Geometry check sheet. Reference: the model listing, model coordinates, mm. A direction names the side the tool comes from. Round coordinates to 2 decimals unless told otherwise and drop trailing zeros. Loops run counter-clockwise (first coordinate to the right, second up) from the corner with the lowest first, then second, coordinate; pieces in that order, holes last.
```python
from build123d import *

# Parameters (mm, degrees)
BOSS_EXTRUDE1_DEPTH = 190
SHELL1_T            = -2
SKETCH3_R           = 17.5
CUT_EXTRUDE2_DEPTH  = 61


with BuildPart() as part:
    # Sketch1 → Boss-Extrude1 (new body, symmetric)
    with BuildSketch(Plane(origin=(0, 0, 0), x_dir=(1, 0, 0), z_dir=(0, 1, 0))):
        with BuildLine():
            Line((-24, -30), (24, -30))
            ThreePointArc((24, -30), (28.242640687, -28.242640687), (30, -24))
            Line((30, -24), (30, 24))
            ThreePointArc((30, 24), (28.242640687, 28.242640687), (24, 30))
            Line((24, 30), (-24, 30))
            ThreePointArc((-24, 30), (-28.242640687, 28.242640687), (-30, 24))
            Line((-30, 24), (-30, -24))
            ThreePointArc((-30, -24), (-28.242640687, -28.242640687), (-24, -30))
        make_face()
    extrude(amount=BOSS_EXTRUDE1_DEPTH, both=True)

    # Shell1
    shell1_openings = [part.faces().sort_by_distance(p)[0] for p in [
        (0, 190, 0),
        (0, -190, 0),
    ]]
    offset(amount=SHELL1_T, openings=shell1_openings, kind=Kind.INTERSECTION)

    # Sketch3 → Cut-Extrude2 (cut, through all)
    with BuildSketch(Plane(origin=(0, 0, -30), x_dir=(-1, 0, 0), z_dir=(0, 0, -1))):
        Circle(SKETCH3_R)
    extrude(amount=-CUT_EXTRUDE2_DEPTH, mode=Mode.SUBTRACT)


solid = part.part
```
1) Access from +Z, -Z, +X, -X, +Y, -Y to the whole of each face (thin tool, end or side, straight path). Record for faces 1 (the face through (28, 3, 0)), 2 (the face through (0, -190, -29)).
Report:
face 1: +Y, -Y
face 2: +Z, -Z, +X, -X, -Y
2) Sectioned sample at D-D, the plane y = 167.5. Record the cut outline in (x, z).
Report:
outline: (-30, -24) arc R6 ccw to (-24, -30) - (24, -30) arc R6 ccw to (30, -24) - (30, 24) arc R6 ccw to (24, 30) - (-24, 30) arc R6 ccw to (-30, 24) - close; hole (-28, -24) arc R4 ccw to (-24, -28) - (24, -28) arc R4 ccw to (28, -24) - (28, 24) arc R4 ccw to (24, 28) - (-24, 28) arc R4 ccw to (-28, 24) - close
3) Scan lines: line 1 along Z through (x, y) = (23.5, 61.5); line 2 along Y through (x, z) = (0, 29). Record each from-to range of solid material in increasing order.
Report:
line 1: z = -30 to -28, 28 to 30
line 2: y = -190 to -17.5, 17.5 to 190
4) Mould release check, pull along X, two halves, no side actions. Record for faces 3 (the face through (21, 3, 28)), 4 (the face through (28.196, 2.66, 28.289)), 5 (the face through (-28.196, 2.66, -28.289)): +X half, -X half, draft (parallel to the pull), parting line (faces both ways), or undercut.
Report:
face 3: undercut
face 4: +X half
face 5: -X half
5) Sectioned sample at B-B, the plane x = 0. Record the cut outline in (y, z).
Report:
outline: (-190, -30) - (-17.5, -30) - (-17.5, -28) - (-190, -28) - close; (-190, 28) - (-17.5, 28) - (-17.5, 30) - (-190, 30) - close; (17.5, -30) - (190, -30) - (190, -28) - (17.5, -28) - close; (17.5, 28) - (190, 28) - (190, 30) - (17.5, 30) - close
6) Sectioned sample at A-A, the plane z = 0.5. Record the cut outline in (x, y).
Report:
outline: (-30, -190) - (-28, -190) - (-28, 190) - (-30, 190) - close; (28, -190) - (30, -190) - (30, 190) - (28, 190) - close
7) Sectioned sample at C-C, the plane y = 0. Record the cut outline in (x, z).
Report:
outline: (-30, -24) arc R6 ccw to (-24, -30) - (-17.5, -30) - (-17.5, -28) - (-24, -28) arc R4 cw to (-28, -24) - (-28, 24) arc R4 cw to (-24, 28) - (-17.5, 28) - (-17.5, 30) - (-24, 30) arc R6 ccw to (-30, 24) - close; (17.5, -30) - (24, -30) arc R6 ccw to (30, -24) - (30, 24) arc R6 ccw to (24, 30) - (17.5, 30) - (17.5, 28) - (24, 28) arc R4 cw to (28, 24) - (28, -24) arc R4 cw to (24, -28) - (17.5, -28) - close
